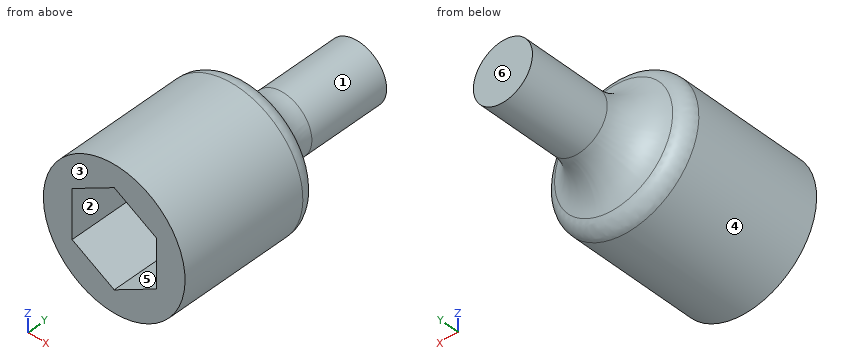
from build123d import *

# Parameters (mm, degrees)
CUT_EXTRUDE1_DEPTH = 15.875
FILLET1_R          = 6.35
FILLET2_R          = 2.54


with BuildPart() as part:
    # Sketch1 → Revolve1 (revolve)
    with BuildSketch(Plane.XY, mode=Mode.PRIVATE) as revolve1_sk:
        Polygon((0, 41.275), (4.6355, 41.275), (4.6355, 22.225), (11.1125, 22.225), (11.1125, 0), (0, 0), align=None)
    revolve(revolve1_sk.sketch.rotate(Axis((0, 0, 0), (0, 1, 0)), 90), axis=Axis((0, 0, 0), (0, 1, 0)))

    # Sketch2 → Cut-Extrude1 (cut)
    with BuildSketch(Plane.XZ):
        Polygon((6.604, 3.812821178), (0, 7.625642355), (-6.604, 3.812821178), (-6.604, -3.812821178), (0, -7.625642355), (6.604, -3.812821178), align=None)
    extrude(amount=-CUT_EXTRUDE1_DEPTH, mode=Mode.SUBTRACT)

    # Fillet1
    fillet1_edges = [part.edges().sort_by_distance(p)[0] for p in [
        (0, 22.225, 4.6355),
    ]]
    fillet(fillet1_edges, radius=FILLET1_R)

    # Fillet2
    fillet2_edges = [part.edges().sort_by_distance(p)[0] for p in [
        (0, 22.225, 11.1125),
    ]]
    fillet(fillet2_edges, radius=FILLET2_R)


solid = part.part
Work out the finished part from the listing and answer in its coordinate system (mm). Face numbers are marked on the shaded views. A direction names the side the tool comes from. Coordinates: 2 decimals unless noted, no trailing zeros. Write each loop counter-clockwise with the first axis right and the second up, starting at its lowest first coordinate (ties: lowest second). Pieces come first, ordered by that corner, then holes. Notation, with made-up numbers: M 67,42.5 L 126,42.5 A26 ccw 126,67.5 Z; hole C 33.5,61 d6. An arc over 180 degrees is marked long. Use one line per item in the form item = value. Start each with the question number.
1. Straight lines are drawn through the part: probe 1 along X at (y, z) = (5.5, 0); probe 2 along Y at (x, z) = (-0.5, 0.75) (3 decimals); probe 3 along Z at (x, y) = (6.25, 13.5). For each, find the intervals that lie inside material, in ascending order. Write a range as from..to.
2. Each of these flat-tipped pins is pushed along its axis until it touches: P1, Ø1, axis at x = -2.5, y = 18, coming from the -Z side; P2, Ø4, axis at x = 3, z = -1.5, coming from the -Y side (3 decimals); P3, Ø2, axis at y = 13.5, z = 6.5, coming from the -X side. Where does it stop, or does it pass through?
3. A tool of negligible diameter and unlimited length cuts with its end or side. For the marked faces 1, 2 and 3, from which of +Z, -Z, +X, -X, +Y, -Y can it reach the whole face along a straight path? Write none if from no direction.
4. The part is cut by section A-A (y = 30). Give the vertices of the cut face in (x, z).
5. The mould has two halves that part along Z. Classify the marked faces 4, 5 and 6: released by +Z, released by -Z, zero draft, split by the parting line, or undercut.
6. The part is cut by section B-B (y = 23.5). Give the vertices of the cut face in (x, z), plus the area to 3 significant figures.
Evaluation:
q1.probe_1 = -11.11..-6.6, 6.6..11.11
q1.probe_2 = 15.875..41.275
q1.probe_3 = -9.19..-4.02, 4.02..9.19
q2.P1 = -10.93
q2.P2 = 15.875
q2.P3 = -9.66
q3.face_1 = +Y
q3.face_2 = -Y
q3.face_3 = +Z, -Z, +X, -X, -Y
q4.outline = C 0,0 d9.27
q5.face_4 = split by the parting line
q5.face_5 = undercut
q5.face_6 = zero draft
q6.outline = C 0,0 d14.34
q6.area = 161 mm^2
